Input: dimensioned drawing with shaded views. Units: mm. Origin: part minimum x, y, z. Round coordinates to 2 decimals unless told otherwise and drop trailing zeros. Order: outer loops, then holes, each group sorted by start corner. A loop starts at its lowest first (then second) coordinate and runs counter-clockwise, first axis right, second up. Notation, with made-up numbers: (70, 72.25) - (74, 72.25) arc R16 cw to (74, 82.25) - close; hole circle Ø8 at (24, 1). An arc over 180 degrees is marked (long way). Put each result on its own line as item: value. Start each with the question number.
(1) Material intervals for L1, parallel to X at y = 1.65, z = 28; L2, parallel to X at y = 0.5, z = 25; L3, parallel to Z at x = 60.5, y = 1.85, sorted ascending. Write a range as [from, to].
(2) Section C-C (x = 125.5). Output: boundary loops of the cut face in (y, z).
(3) Section A-A (z = 28). Output: boundary loops of the cut face in (x, y).
(4) Section B-B (y = 2.4). Output: boundary loops of the cut face in (x, z), and give its area (3 significant figures).
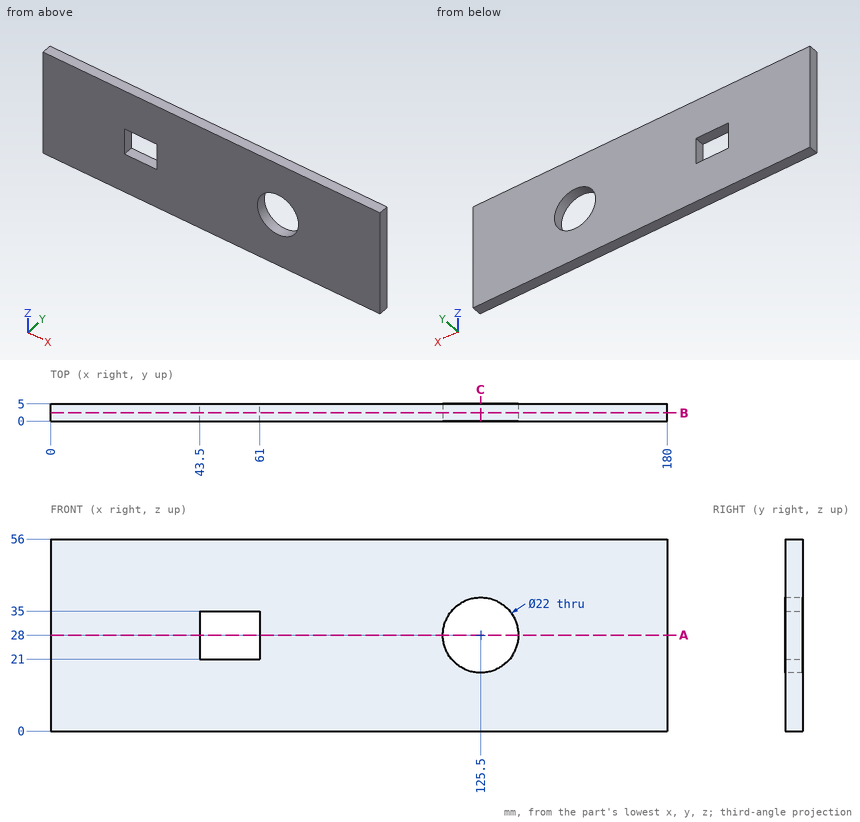
Checks:
1. L1: x = [0, 43.5], [61, 114.5], [136.5, 180]
1. L2: x = [0, 43.5], [61, 114.92], [136.08, 180]
1. L3: z = [0, 21], [35, 56]
2. outline: (0, 0) - (5, 0) - (5, 17) - (0, 17) - close; (0, 39) - (5, 39) - (5, 56) - (0, 56) - close
3. outline: (0, 0) - (43.5, 0) - (43.5, 5) - (0, 5) - close; (61, 0) - (114.5, 0) - (114.5, 5) - (61, 5) - close; (136.5, 0) - (180, 0) - (180, 5) - (136.5, 5) - close
4. outline: (0, 0) - (180, 0) - (180, 56) - (0, 56) - close; hole (43.5, 21) - (61, 21) - (61, 35) - (43.5, 35) - close; hole circle Ø22 at (125.5, 28)
4. area: 9,450 mm²
